```python
from build123d import *

# Parameters (mm, degrees)
F0_W     = 40
F0_H     = 30
F1_DEPTH = 50
F2_R     = 12.5
F3_DEPTH = 20
F4_R     = 2
F5_SIZE  = 5


with BuildPart() as f1:
    # F0 (on Front) → F1 (new body)
    with BuildSketch(Plane.XZ):
        Rectangle(F0_W, F0_H)
    extrude(amount=F1_DEPTH)

    # F2 (on face) → F3 (join)
    with BuildSketch(Plane.XZ.offset(50)):
        Circle(F2_R)
    extrude(amount=F3_DEPTH)

    # F4
    f4_edges = [f1.edges().sort_by_distance(p)[0] for p in [
        (-12.5, -70, 0),
    ]]
    fillet(f4_edges, radius=F4_R)

    # F5
    f5_edges = [f1.edges().sort_by_distance(p)[0] for p in [
        (-20, -25, 15),
        (20, -25, 15),
    ]]
    chamfer(f5_edges, length=F5_SIZE)


solid = f1.part
```
Build history of the part. All positions in model axes, mm. A direction names the side the tool comes from. Give positions to 0.01 mm unless a question says otherwise; leave off trailing zeros. Order: outer loops, then holes, each group sorted by start corner. A loop starts at its lowest first (then second) coordinate and runs counter-clockwise, first axis right, second up. Notation, with made-up numbers: M 52.5,37 L 105.5,37 A8 ccw 105.5,50 Z; hole C 56.25,57.5 d3. An arc over 180 degrees is marked long. Return JSON: item names as keys, results as strings.
Q1. Flat gauge pins, fed straight in: pin 1 (2 mm diameter, centred on x = -10, y = -51.5, fed in from -Z); pin 2 (6 mm diameter, centred on x = -12.5, y = -60.5, fed in from -Z); pin 3 (3 mm diameter, centred on y = -57.5, z = -8.5, fed in from -X). Where does each tip first touch, or does it go through?
Answer list:
{"pin 1": "stops at z = -8.67", "pin 2": "stops at z = -8.12", "pin 3": "stops at x = -10.36"}
Q2. Band-saw the part on C-C (y = -9). Give the cut face in (x, z).
Answer list:
{"outline": "M -20,-15 L 20,-15 L 20,10 L 15,15 L -15,15 L -20,10 Z"}
Q3. Band-saw the part on B-B (x = 0). Give the cut face in (y, z), then the cut area to 3 significant figures.
Answer list:
{"outline": "M -70,-10.5 A2 ccw -68,-12.5 L -50,-12.5 L -50,-15 L 0,-15 L 0,15 L -50,15 L -50,12.5 L -68,12.5 A2 ccw -70,10.5 Z", "area": "2,000 mm^2"}
Q4. 3-axis set-ups, long thin cutter, end or side, ignore diameter. For faces 1 (the face through (0, -50, -13)), 2 (the face through (0, -70, 0)): which of +Z, -Z, +X, -X, +Y, -Y reach the whole face in a straight line?
Answer list:
{"face 1": "-Y", "face 2": "+Z, -Z, +X, -X, -Y"}
Q5. Band-saw the part on A-A (z = 0). Give the cut face in (x, y).
Answer list:
{"outline": "M -20,-50 L -12.5,-50 L -12.5,-68 A2 ccw -10.5,-70 L 10.5,-70 A2 ccw 12.5,-68 L 12.5,-50 L 20,-50 L 20,0 L -20,0 Z"}
Q6. Wall check: probe 1 along Y at (x, z) = (-15.5, -1.75); probe 2 along Z at (x, y) = (0, -62); probe 3 along X at (y, z) = (-36, 11). Give the ranges that are in metal, low to high. Write a range as from..to.
Answer list:
{"probe 1": "y = -50..0", "probe 2": "z = -12.5..12.5", "probe 3": "x = -19..19"}
Q7. Band-saw the part on D-D (x = 16.5). Give the cut face in (y, z), then the cut area to 4 significant figures.
Answer list:
{"outline": "M -50,-15 L 0,-15 L 0,13.5 L -50,13.5 Z", "area": "1,425 mm^2"}
